```python
from build123d import *

# Parameters (mm, degrees)
SALIENTE_EXTRUIR1_DEPTH    = 29
CORTAR_EXTRUIR7_DEPTH      = 32.080540536
CORTAR_EXTRUIR7_DEPTH_BACK = 32.080540536
CROQUIS5_W                 = 6.75461664
CROQUIS5_H                 = 6
CORTAR_EXTRUIR8_DEPTH      = 32.701734968
CORTAR_EXTRUIR8_DEPTH_BACK = 32.701734968
CROQUIS9_W                 = 17.209263494
CROQUIS9_H                 = 6
REDONDEO3_R                = 2.5


with BuildPart() as part:
    # Croquis2 → Saliente-Extruir1 (new body)
    with BuildSketch(Plane.XY):
        with BuildLine():
            Line((-3, -4), (-3, -10))
            Line((-3, -10), (3, -10))
            Line((3, -10), (3, -4))
            ThreePointArc((3, -4), (0, 5), (-3, -4))
        make_face()
    extrude(amount=SALIENTE_EXTRUIR1_DEPTH)

    # Croquis5 → Cortar-Extruir7 (cut, two sides: drawn at the far end of the back side and taken through both)
    with BuildSketch(Plane(origin=(0, 0, 0), x_dir=(0, 0, -1), z_dir=(1, 0, 0)).offset(-CORTAR_EXTRUIR7_DEPTH_BACK)):
        with Locations((-25.62269168, -7)):
            Rectangle(CROQUIS5_W, CROQUIS5_H)
    extrude(amount=CORTAR_EXTRUIR7_DEPTH + CORTAR_EXTRUIR7_DEPTH_BACK, mode=Mode.SUBTRACT)

    # Croquis9 → Cortar-Extruir8 (cut, two sides: drawn at the far end of the back side and taken through both)
    with BuildSketch(Plane(origin=(3, 0, 0), x_dir=(0, 0, -1), z_dir=(1, 0, 0)).offset(-CORTAR_EXTRUIR8_DEPTH_BACK)):
        with Locations((-8.604631747, -7)):
            Rectangle(CROQUIS9_W, CROQUIS9_H)
    extrude(amount=CORTAR_EXTRUIR8_DEPTH + CORTAR_EXTRUIR8_DEPTH_BACK, mode=Mode.SUBTRACT)

    # Redondeo3
    # the kernel refuses this fillet: 2.5 mm, written as the material it takes off along each edge
    with BuildSketch(Plane(origin=(9.25, -4, 29), x_dir=(0, 0, -1), z_dir=(-1, 0, 0))) as redondeo3_piece_1:
        with BuildLine():
            CenterArc((REDONDEO3_R, -REDONDEO3_R), REDONDEO3_R, 90, 90)
            Line((0, -REDONDEO3_R), (0, 0))
            Line((0, 0), (REDONDEO3_R, 0))
        make_face()
    extrude(amount=18.5, mode=Mode.SUBTRACT)
    with BuildSketch(Plane(origin=(9.25, -4, 0), x_dir=(0, 0, 1), z_dir=(-1, 0, 0))) as redondeo3_piece_2:
        with BuildLine():
            CenterArc((REDONDEO3_R, REDONDEO3_R), REDONDEO3_R, 180, 90)
            Line((0, REDONDEO3_R), (0, 0))
            Line((0, 0), (REDONDEO3_R, 0))
        make_face()
    extrude(amount=18.5, mode=Mode.SUBTRACT)
    with BuildSketch(Plane(origin=(0, 0, 0), x_dir=(0.0031415874858798706, -0.9999950652018581, 0), z_dir=(-0.9999950652018581, -0.0031415874858798706, 0))) as redondeo3_piece_3:
        with BuildLine():
            CenterArc((5 - REDONDEO3_R, REDONDEO3_R), REDONDEO3_R, 270, 90)
            Line((5 - REDONDEO3_R, 0), (5, 0))
            Line((5, 0), (5, REDONDEO3_R))
        make_face()
    revolve(axis=Axis((0, 0, 0), (0, 0, 1)), revolution_arc=359.64, mode=Mode.SUBTRACT)
    with BuildSketch(Plane(origin=(0, 0, 29), x_dir=(0.0031415874858798706, -0.9999950652018581, 0), z_dir=(-0.9999950652018581, -0.0031415874858798706, 0))) as redondeo3_piece_4:
        with BuildLine():
            CenterArc((5 - REDONDEO3_R, -REDONDEO3_R), REDONDEO3_R, 0, 90)
            Line((5 - REDONDEO3_R, 0), (5, 0))
            Line((5, 0), (5, -REDONDEO3_R))
        make_face()
    revolve(axis=Axis((0, 0, 29), (0, 0, 1)), revolution_arc=359.64, mode=Mode.SUBTRACT)


solid = part.part
```
Design review of the part built by this model. Coordinates are the model's own, in mm. A direction names the side the tool comes from. Give positions to 0.01 mm unless a question says otherwise; leave off trailing zeros. Loops run counter-clockwise (first coordinate to the right, second up) from the corner with the lowest first, then second, coordinate; pieces in that order, holes last. Notation, with made-up numbers: (15.5, -6) -> (69.5, -6) arc R23 ccw to (69.5, 4) -> close; hole circle Ø6 at (33, -23). An arc over 180 degrees is marked (long way). One line per item, written item: value.
Q1. We need section B-B on z = 10.5. Give the boundary of the cut face in (x, y), and give its area (3 significant figures).
Numbers:
outline: (-3, -4) -> (3, -4) arc R5 ccw (long way) to start
area: 74.5 mm^2
Q2. For pin 1 Ø5 at (x, y) = (-3, -4) entering from -Z; pin 2 Ø5 at (x, z) = (-0.5, 13.5) entering from -Y; pin 3 Ø1.5 at (x, z) = (1.5, 7) entering from +Y, all flat-tipped, find the tip position at first contact; note any pin that passes through.
Numbers:
pin 1: stops at z = 0.01
pin 2: stops at y = -4
pin 3: stops at y = 4.94
Q3. Machinability: for faces 1 (the flat face through (0, -4, 24)), 2 (the flat face through (0, -7, 17.209)), 3 (the flat face through (-3, -7, 20)), 4 (the flat face through (0, -10, 20)), 5 (the flat face through (3, -7, 20)), which of the approach directions +Z, -Z, +X, -X, +Y, -Y give a long, thin tool a straight path to every point of the face, cutting with its end or side? Answer none if there is none.
Numbers:
face 1: +Z, +X, -X, -Y
face 2: -Z, +X, -X, -Y
face 3: +Z, -Z, -X, -Y
face 4: +Z, -Z, +X, -X, -Y
face 5: +Z, -Z, +X, -Y
Q4. For L1, parallel to Z at x = 1.75, y = -6; L2, parallel to Y at x = -4, z = 24.25; L3, parallel to X at y = 4.25, z = 18.5, list the stretches that pass through material, from the lowest coordinate up.
Numbers:
L1: z = 17.21 to 22.25
L2: y = -3 to 3
L3: x = -2.63 to 2.63
Q5. We need section A-A on z = 18.75. Give the boundary of the cut face in (x, y).
Numbers:
outline: (-3, -10) -> (3, -10) -> (3, -4) arc R5 ccw (long way) to (-3, -4) -> close
